from build123d import *

# Parameters (mm, degrees)
SKETCH1_W           = 80
SKETCH1_H           = 80
BOSS_EXTRUDE1_DEPTH = 30
SKETCH2_W           = 61
SKETCH2_H           = 10.2
CUT_EXTRUDE1_DEPTH  = 65.031242374
SKETCH3_W           = 40
SKETCH3_H           = 25
CUT_EXTRUDE2_DEPTH  = 20
SKETCH4_R           = 3.5
CUT_EXTRUDE3_DEPTH  = 61
SKETCH5_R           = 3.5
CUT_EXTRUDE4_DEPTH  = 95.339811321
SKETCH6_R           = 7.5
CUT_EXTRUDE5_DEPTH  = 65.031242374


with BuildPart() as part:
    # Sketch1 → Boss-Extrude1 (new body)
    with BuildSketch(Plane.XY):
        Rectangle(SKETCH1_W, SKETCH1_H)
    extrude(amount=BOSS_EXTRUDE1_DEPTH)

    # Sketch2 → Cut-Extrude1 (cut, through all)
    with BuildSketch(Plane.XY.offset(30)):
        with Locations((0, 31.9)):
            Rectangle(SKETCH2_W, SKETCH2_H)
    extrude(amount=-CUT_EXTRUDE1_DEPTH, mode=Mode.SUBTRACT)

    # Sketch3 → Cut-Extrude2 (cut)
    with BuildSketch(Plane(origin=(0, 0, 0), x_dir=(-1, 0, 0), z_dir=(0, 0, -1))):
        with Locations((0, -27.5)):
            Rectangle(SKETCH3_W, SKETCH3_H)
    extrude(amount=-CUT_EXTRUDE2_DEPTH, mode=Mode.SUBTRACT)

    # Sketch4 → Cut-Extrude3 (cut, through all)
    with BuildSketch(Plane(origin=(0, 0, 20), x_dir=(-1, 0, 0), z_dir=(0, 0, -1))):
        with Locations((0, -25)):
            Circle(SKETCH4_R)
    extrude(amount=-CUT_EXTRUDE3_DEPTH, mode=Mode.SUBTRACT)

    # Sketch5 → Cut-Extrude4 (cut, through all)
    with BuildSketch(Plane(origin=(40, 0, 0), x_dir=(0, 0, -1), z_dir=(1, 0, 0))):
        with Locations((-15, 33.619017373)):
            Circle(SKETCH5_R)
    extrude(amount=-CUT_EXTRUDE4_DEPTH, mode=Mode.SUBTRACT)

    # Sketch6 → Cut-Extrude5 (cut, through all)
    with BuildSketch(Plane.XY.offset(30)):
        with Locations((29.056312598, 16)):
            Circle(SKETCH6_R)
    extrude(amount=-CUT_EXTRUDE5_DEPTH, mode=Mode.SUBTRACT)


solid = part.part
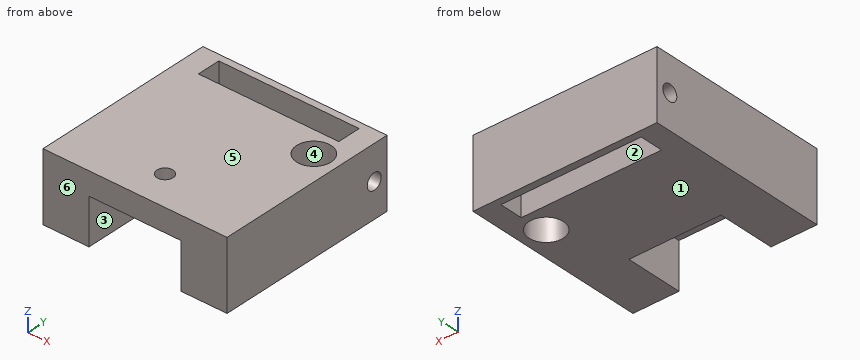
Verification items for the finished model (mm, model axes). Face numbers are marked on the shaded views. A direction names the side the tool comes from. Give positions to 0.01 mm unless a question says otherwise; leave off trailing zeros. Loops run counter-clockwise (first coordinate to the right, second up) from the corner with the lowest first, then second, coordinate; pieces in that order, holes last.
1) Sectioned sample at B-B, the plane x = 0. Enter the section's corners in (y, z), then the cut area to 3 significant figures.
2) Sectioned sample at D-D, the plane y = 16. Enter the section's corners in (x, z), then the cut area to 3 significant figures.
3) Depth check by flat-ended pin: pin 1 Ø17 at (x, y) = (29.06, 16) entering from +Z; pin 2 Ø4 at (x, z) = (-4.5, 3.5) entering from -Y; pin 3 Ø7.5 at (x, y) = (7, -30.5) entering from -Z. Enter the tip coordinate at first touch or a pass-through.
4) Thickness scan on line 1 along Y through (x, z) = (0, 27); line 2 along Y through (x, z) = (-4.5, 12.25); line 3 along X through (y, z) = (-31.5, 14.5). Record the ranges inside material, lowest first.
5) Sectioned sample at C-C, the plane y = -25. Enter the section's corners in (x, z).
6) Set-up check for the marked faces 1, 2 and 3: record each of +Z, -Z, +X, -X, +Y, -Y from which the full face is reachable in a straight line by a thin tool's end or side.
7) Sectioned sample at A-A, the plane x = -26. Enter the section's corners in (y, z).
8) Draft check along Y on the marked faces 4, 5 and 6. Enter one of: pulls with the +Y half, pulls with the -Y half, needs draft (parallel to the pull), parting line crosses it, or undercut.
Answers:
1. outline: (-40, 20) - (-28.5, 20) - (-28.5, 30) - (-40, 30) - close; (-21.5, 20) - (-15, 20) - (-15, 0) - (26.8, 0) - (26.8, 30) - (-21.5, 30) - close; (37, 0) - (40, 0) - (40, 30) - (37, 30) - (37, 15.9) arc R3.5 cw to (37, 14.1) - close
1. area: 1,520 mm2
2. outline: (-40, 0) - (21.56, 0) - (21.56, 30) - (-40, 30) - close; (36.56, 0) - (40, 0) - (40, 30) - (36.56, 30) - close
2. area: 1,950 mm2
3. pin 1: stops at z = 30
3. pin 2: stops at y = -15
3. pin 3: stops at z = 20
4. line 1: y = -40 to -28.5, -21.5 to 26.8, 37 to 40
4. line 2: y = -15 to 26.8, 37 to 40
4. line 3: x = -40 to -20, 20 to 40
5. outline: (-40, 0) - (-20, 0) - (-20, 20) - (-3.5, 20) - (-3.5, 30) - (-40, 30) - close; (3.5, 20) - (20, 20) - (20, 0) - (40, 0) - (40, 30) - (3.5, 30) - close
6. face 1: -Z, +X, -X, +Y, -Y
6. face 2: +Z, -Z
6. face 3: -Z, -Y
7. outline: (-40, 0) - (26.8, 0) - (26.8, 30) - (-40, 30) - close; (37, 0) - (40, 0) - (40, 30) - (37, 30) - (37, 15.9) arc R3.5 cw to (37, 14.1) - close
8. face 4: undercut
8. face 5: needs draft
8. face 6: pulls with the -Y half
